Autodesk Inventor part; units mm, degrees
ref_plane "YZ Plane" through (0, 0, 0) normal (1, 0, 0) x (0, 1, 0)
ref_plane "XZ Plane" through (0, 0, 0) normal (0, 1, 0) x (-1, 0, 0)
ref_plane "XY Plane" through (0, 0, 0) normal (0, 0, 1) x (1, 0, 0)
sketch "스케치1" plane through (0, 0, 0) normal (0, 0, 1) x (1, 0, 0)
  line L0 (18.1059, -15.875) -> (-18.1059, -15.875)
  line L1 (-18.1059, -15.875) -> (-18.1059, 15.875)
  line L2 (-18.1059, 15.875) -> (18.1059, 15.875)
  line L3 (18.1059, 15.875) -> (18.1059, -15.875)
  line L4 (18.1059, -15.875) -> (-18.1059, 15.875) construction
  line L5 (-18.1059, -15.875) -> (18.1059, 15.875) construction
  point P0 (0, 0)
extrude "돌출1" add sketch "스케치1" along normal blind 30
sketch "스케치2" plane through (-18.1059, 15.875, 0) normal (0, 1, 0) x (1, 0, 0)
  line L0 (0, -30) -> (36.2119, -30)
  line L1 (36.2119, 0) -> (36.2119, -30)
  line L2 (4.0585, -30) -> (36.2119, -30)
  line L3 (36.2119, -30) -> (36.2119, -19.9659)
  line L4 (36.2119, -19.9659) -> (4.0585, -19.9659)
  line L5 (4.0585, -19.9659) -> (4.0585, -30)
  line L6 (36.2119, 0) -> (0, 0)
  line L7 (4.0585, 0) -> (36.2119, 0)
  line L8 (36.2119, 0) -> (36.2119, -10.034)
  line L9 (36.2119, -10.034) -> (4.0585, -10.034)
  line L10 (4.0585, -10.034) -> (4.0585, 0)
  point P0 (18.1059, 0)
  dimension "d2" = 10.034
extrude "돌출2" cut sketch "스케치2" against normal blind 28
sketch "스케치3" plane through (-18.1059, 15.875, 30) normal (0, 1, 0) x (1, 0, 0)
  line L0 (4.0585, 10.0341) -> (36.2119, 10.0341)
  line L1 (36.2119, 30) -> (36.2119, 0)
  line L2 (31.9669, 10.0341) -> (36.2119, 10.0341)
  line L3 (36.2119, 10.0341) -> (36.2119, 20.0064)
  line L4 (36.2119, 20.0064) -> (31.9669, 20.0064)
  line L5 (31.9669, 20.0064) -> (31.9669, 10.0341)
  point P0 (18.1059, 30)
extrude "돌출3" cut sketch "스케치3" against normal blind 50
sketch "스케치4" plane through (-14.0475, -12.125, 19.9659) normal (0, 0, 1) x (1, 0, 0)
  line L0 (0, 0) -> (22.1415, 0)
  line L1 (22.1415, 0) -> (22.1415, 23.4499)
  line L2 (22.1415, 23.4499) -> (0, 23.4499)
  line L3 (0, 23.4499) -> (0, 0)
  point P0 (14.0475, 12.125)
extrude "돌출4" cut sketch "스케치4" against normal blind 50
sketch "스케치5" plane through (-14.0475, 15.875, 30) normal (1, 0, 0) x (0, 0, -1)
  circle A0 centre (5.0001, -4.0724) radius 2.0226
  circle A1 centre (25.7482, -4.0724) radius 2.1705
  point P0 (30, -15.875)
extrude "돌출5" cut sketch "스케치5" against normal blind 50
sketch "스케치6" plane through (-18.1059, -12.125, 0) normal (0, 1, 0) x (1, 0, 0)
  circle A0 centre (31.4326, -4.8571) radius 2.5553
  circle A1 centre (31.4326, -25.7502) radius 2.6688
  point P0 (18.1059, 0)
extrude "돌출6" cut sketch "스케치6" against normal blind 50
sketch "스케치7" plane through (-18.1059, 15.875, 30) normal (0, 1, 0) x (1, 0, 0)
  circle A0 centre (11.6135, 14.7451) radius 2.7078
  point P0 (18.1059, 30)
extrude "돌출7" cut sketch "스케치7" against normal blind 20
sketch "스케치8" plane through (13.861, 15.875, 19.9659) normal (1, 0, 0) x (0, 0, -1)
  circle A0 centre (4.9416, -23.8738) radius 2.5891
  point P0 (19.9659, -15.875)
extrude "돌출8" cut sketch "스케치8" against normal blind 20
fillet "모깎기1" radius 6 1 edges at (13.861, 15.875, 15)
sketch "스케치9" plane through (-14.0475, 15.875, 19.9659) normal (0, 1, 0) x (1, 0, 0)
  line L0 (-4.0585, 19.9659) -> (-4.0585, -10.0341)
  line L1 (-4.0585, 9.9335) -> (21.8906, 9.9335)
  line L2 (21.8906, 9.9335) -> (21.8906, -0.0015)
  line L3 (21.8906, -0.0015) -> (-4.0585, -0.0015)
  line L4 (-4.0585, -0.0015) -> (-4.0585, 9.9335)
  point P0 (14.0475, 19.9659)
  point P1 (-4.0585, 15.9659)
  point P2 (-4.0585, -6.0341)
sketch "스케치10" plane through (-14.0475, 15.875, 19.9659) normal (0, 1, 0) x (1, 0, 0)
  point P0 (14.0475, 19.9659)
sketch "스케치11" plane through (-18.1059, 15.875, 30) normal (0, 1, 0) x (1, 0, 0)
  line L0 (0, 30) -> (0, 0)
  line L1 (4.0585, 0) -> (4.0585, 30)
  line L2 (0, 30) -> (4.0585, 30)
  line L3 (4.0585, 30) -> (4.0585, 19.8806)
  line L4 (4.0585, 19.8806) -> (0, 19.8806)
  line L5 (0, 19.8806) -> (0, 30)
  line L6 (36.2119, 0) -> (4.0585, 0)
  line L7 (0, 10.0954) -> (4.0585, 10.0954)
  line L8 (4.0585, 10.0954) -> (4.0585, 0)
  line L9 (4.0585, 0) -> (0, 0)
  line L10 (0, 0) -> (0, 10.0954)
  point P0 (18.1059, 30)
extrude "돌출9" add sketch "스케치11" along normal blind 5 contours L2 L1 L4 L0 | L7 L1 L9 L0
fillet "모깎기3" radius 4 5 edges at (-16.0767, 20.875, 30) (-16.0767, 20.875, 0) (18.1059, -14, 30) (18.1059, -14, 0) (-18.1059, -15.875, 15)
properties part number "240510_3Dsketch04"
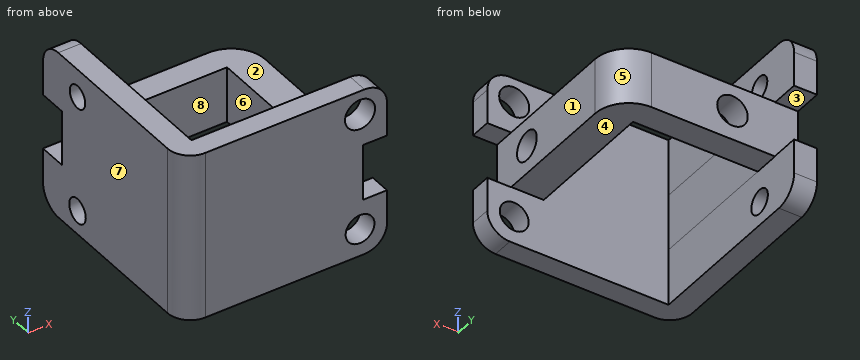
Source: CAD feature listing. Evaluate the final solid. Frame: model axes, mm. Face numbers are marked on the shaded views. A direction names the side the tool comes from. Coordinates: 2 decimals unless noted, no trailing zeros. Write each loop counter-clockwise with the first axis right and the second up, starting at its lowest first coordinate (ties: lowest second). Pieces come first, ordered by that corner, then holes. Notation, with made-up numbers: M -37.75,-17.5 L -11.75,-17.5 A19 ccw -11.75,19.5 Z; hole C -16.5,89 d9. An arc over 180 degrees is marked long. Answer as a JSON object with one key per item and string values.
1. Cut plane D-D on x = -5.5. Output: boundary loops of the cut face in (y, z) (3 decimals).
Evaluation:
{"outline": "M -15.875,0 L -12.125,0 L -12.125,30 L -15.875,30 Z; M 11.325,10.034 L 15.875,10.034 L 15.875,12.736 L 11.325,12.736 Z; M 11.325,17.774 L 15.875,17.774 L 15.875,19.966 L 11.325,19.966 Z"}
2. Cut plane A-A on y = 3. Output: boundary loops of the cut face in (x, z).
Evaluation:
{"outline": "M -18.11,0 L -14.05,0 L -14.05,10.03 L -14.05,30 L -18.11,30 Z; M 8.09,10.03 L 13.86,10.03 L 13.86,19.97 L 8.09,19.97 Z"}
3. Ray query, L1, parallel to Y at x = 4, z = 11.75 (3 decimals); L2, parallel to X at y = -10, z = 16.75; L3, parallel to X at y = -3, z = 20.5. Return the intervals inside material, ascending.
Evaluation:
{"L1": "-15.875 to -12.125, 11.325 to 15.875", "L2": "-18.11 to -14.05, 8.09 to 13.86", "L3": "-18.11 to -14.05"}
4. Draft query along X for the marked faces 5, 6, 7 and 8. Return one class per face: released by +X, released by -X, zero draft, split by the parting line, or undercut.
Evaluation:
{"face 5": "released by +X", "face 6": "undercut", "face 7": "released by -X", "face 8": "undercut"}
5. Access query for the marked faces 1, 2, 3 and 4. Directions: +Z, -Z, +X, -X, +Y, -Y. A direction counts if a zero-diameter tool reaches every point of the face in a straight line with its end or side. Return the directions, or none.
Evaluation:
{"face 1": "+X, +Y, -Y", "face 2": "+Z, +X, +Y", "face 3": "+X, -X, +Y", "face 4": "-Z, +X, +Y"}
6. Cut plane C-C on z = 16.5. Output: boundary loops of the cut face in (x, y) (1 decimal), plus the area to 3 significant figures.
Evaluation:
{"outline": "M -18.1,-11.9 A4 ccw -14.1,-15.9 L 13.9,-15.9 L 13.9,-10.1 L 8.1,-10.1 L 8.1,-12.1 L -14,-12.1 L -14,11.3 L -8.9,11.3 L -8.9,15.9 L -18.1,15.9 Z; M -4.1,11.3 L 8.1,11.3 L 8.1,-5.9 L 13.9,-5.9 L 13.9,9.9 A6 ccw 7.9,15.9 L -4.1,15.9 Z", "area": "438 mm^2"}
7. Cut plane B-B on x = 3. Output: boundary loops of the cut face in (y, z) (3 decimals), plus the area to 3 significant figures.
Evaluation:
{"outline": "M -15.875,0 L -12.125,0 L -12.125,30 L -15.875,30 Z; M 11.325,10.034 L 15.875,10.034 L 15.875,19.966 L 11.325,19.966 Z", "area": "158 mm^2"}
8. Contact query for flat-ended pins moving along their axis: P1, Ø1.9, axis at x = 17, y = -13, coming from the +Z side; P2, Ø2, axis at x = 3.5, y = 13, coming from the +Z side; P3, Ø9, axis at x = -3.5, z = 15.5, coming from the +Y side (3 decimals). Output: stop coordinate, or through.
Evaluation:
{"P1": "z = 29.5", "P2": "z = 19.97", "P3": "y = 15.875"}
